Can you work these out from the model? Positions are in its coordinate system, mm. Face numbers are marked on the shaded views. Coordinates: 2 decimals unless noted, no trailing zeros. Loops run counter-clockwise (first coordinate to the right, second up) from the corner with the lowest first, then second, coordinate; pieces in that order, holes last. Notation, with made-up numbers: M 5,8 L 64,8 A18 cw 64,19 Z; hole C -9,57.5 d11. An arc over 180 degrees is marked long. Return JSON: item names as keys, results as strings. Group by question number.
```python
from build123d import *

# Parameters (mm, degrees)
F0_R     = 9
F1_DEPTH = 1.5
F3_R     = 9
F4_DEPTH = 10.5
F5_R     = 6
F6_DEPTH = 2
F7_R     = 7
F8_DEPTH = 9
F9_SIZE  = 0.49999


# Not quite as in the source:
# - a fillet or chamfer that OpenCascade refuses, or shapes differently, is made with other operations: its cross-section is extruded or revolved along the edge and cut away or added
# - a fillet or chamfer is up to 0.001 mm smaller than in the source, because OpenCascade refuses the exact size


with BuildPart() as f1:
    # F0 (on Front) → F1 (new body)
    with BuildSketch(Plane.XZ):
        Circle(F0_R)
    extrude(amount=F1_DEPTH)

    # F2: fillet of radius 9 on 1 edges, made by hand

    # F2_s1 → F2_t2 (revolve, cut)
    with BuildSketch(Plane.XY):
        with BuildLine():
            ThreePointArc((9, 0), (6.6231390258, -1.1168439698), (4.0250628145, -1.5))
            Line((4.0250628145, -1.5), (4.0250628145, -1.68))
            Line((4.0250628145, -1.68), (9, -1.68))
            Line((9, -1.68), (9.18, -1.5))
            ThreePointArc((9.18, -1.5), (9.18, -0.75), (9.0994987437, -0.15))
            Line((9.0994987437, -0.15), (9, 0))
        make_face()
    revolve(axis=Axis((0, -1.5, 0), (0, -1, 0)), mode=Mode.SUBTRACT)

    # F3 (on face) → F4 (join)
    with BuildSketch(Plane(origin=(0, 0, 0), x_dir=(-1, 0, 0), z_dir=(0, 1, 0))):
        Circle(F3_R)
    extrude(amount=F4_DEPTH)

    # F5 (on face) → F6 (join)
    with BuildSketch(Plane(origin=(0, 10.5, 0), x_dir=(-1, 0, 0), z_dir=(0, 1, 0))):
        Circle(F5_R)
    extrude(amount=F6_DEPTH)

    # F7 (on face) → F8 (join)
    with BuildSketch(Plane(origin=(0, 12.5, 0), x_dir=(-1, 0, 0), z_dir=(0, 1, 0))):
        Circle(F7_R)
    extrude(amount=F8_DEPTH)

    # F9 (size 0.5 in the source; OpenCascade refuses exactly that, so slightly less here)
    f9_edges = [f1.edges().sort_by_distance(p)[0] for p in [
        (6, 12.5, 0),
        (6, 10.5, 0),
        (9, 10.5, 0),
        (7, 12.5, 0),
        (7, 21.5, 0),
    ]]
    chamfer(f9_edges, length=F9_SIZE)


solid = f1.part
```
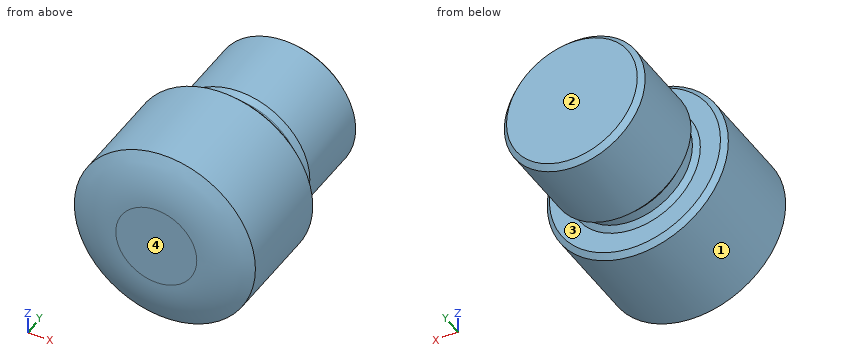
1) For pin 1 (8 mm diameter, centred on x = -3, y = 16.5, fed in from -Z); pin 2 (1 mm diameter, centred on y = 14, z = -3, fed in from +X); pin 3 (3 mm diameter, centred on y = 8.5, z = -4.5, fed in from +X), each with a flat end and sliding along its axis, tell me the tip position at first contact or that it passes through.
2) If I drill on line 1 (Y direction, x = 2, z = 6.5); line 2 (X direction, y = 5.5, z = -4.5); line 3 (Z direction, x = 8.25, y = 0.5), over which ranges is the centre line in solid material (lowest first)? Write a range as from..to.
3) If we mould it in two halves opening along Y, with no side actions, what happens to the marked faces 1, 2, 3 and 4? For each: +Y half, -Y half, draft (parallel to the pull), parting line (faces both ways), or undercut.
4) Suppose I cut it at A-A, the plane y = 17.5. List the corners of the cut face in (x, z) for me, then the cut area to 3 significant figures.
5) Suppose I cut it at B-B, the plane y = 4.5. List the corners of the cut face in (x, z) for me, then the cut area to 3 significant figures.
Returned:
{
 "1": {"pin 1": "stops at z = -7", "pin 2": "stops at x = 6.54", "pin 3": "stops at x = 8.49"},
 "2": {"line 1": "y = -1.06..10.5, 12.8..21.2", "line 2": "x = -7.79..7.79", "line 3": "z = -3.6..3.6"},
 "3": {"face 1": "draft", "face 2": "+Y half", "face 3": "undercut", "face 4": "-Y half"},
 "4": {"outline": "C 0,0 d14", "area": "154 mm²"},
 "5": {"outline": "C 0,0 d18", "area": "254 mm²"}
}
